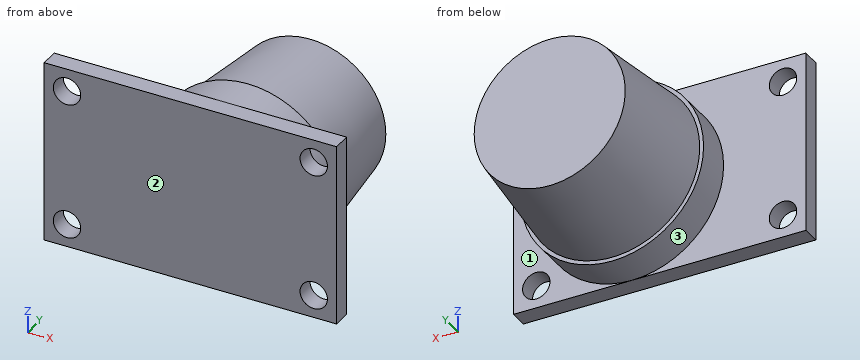
```python
from build123d import *

# Parameters (mm, degrees)
CROQUIS1_W              = 32
CROQUIS1_H              = 20
CROQUIS1_R              = 1.5
SALIENTE_EXTRUIR1_DEPTH = 2
CROQUIS2_R              = 10
SALIENTE_EXTRUIR2_DEPTH = 16.5
SALIENTE_EXTRUIR2_TAPER = 6
CROQUIS4_R              = 10
SALIENTE_EXTRUIR3_DEPTH = 4


with BuildPart() as part:
    # Croquis1 → Saliente-Extruir1 (new body)
    with BuildSketch(Plane(origin=(0, 0, 0), x_dir=(1, 0, 0), z_dir=(0, 1, 0))):
        Rectangle(CROQUIS1_W, CROQUIS1_H)
        with Locations(Location((-13.5, 7.5, 0), (0, 0, 270))):
            Circle(CROQUIS1_R, mode=Mode.SUBTRACT)
        with Locations(Location((13.5, 7.5, 0), (0, 0, 270))):
            Circle(CROQUIS1_R, mode=Mode.SUBTRACT)
        with Locations(Location((-13.5, -7.5, 0), (0, 0, 270))):
            Circle(CROQUIS1_R, mode=Mode.SUBTRACT)
        with Locations(Location((13.5, -7.5, 0), (0, 0, 270))):
            Circle(CROQUIS1_R, mode=Mode.SUBTRACT)
    extrude(amount=SALIENTE_EXTRUIR1_DEPTH)

    # Croquis2 → Saliente-Extruir2 (add)
    with BuildSketch(Plane(origin=(0, 2, 0), x_dir=(1, 0, 0), z_dir=(0, 1, 0))):
        with Locations((3, 0)):
            Circle(CROQUIS2_R)
    extrude(amount=SALIENTE_EXTRUIR2_DEPTH, taper=SALIENTE_EXTRUIR2_TAPER)

    # Croquis4 → Saliente-Extruir3 (add)
    with BuildSketch(Plane(origin=(0, 2, 0), x_dir=(1, 0, 0), z_dir=(0, 1, 0))):
        with Locations(Location((3, 0, 0), (0, 0, 270))):
            Circle(CROQUIS4_R)
    extrude(amount=SALIENTE_EXTRUIR3_DEPTH)


solid = part.part
```
Can you work these out from the model? Positions are in its coordinate system, mm. Face numbers are marked on the shaded views. A direction names the side the tool comes from. Give positions to 0.01 mm unless a question says otherwise; leave off trailing zeros. Write each loop counter-clockwise with the first axis right and the second up, starting at its lowest first coordinate (ties: lowest second). Pieces come first, ordered by that corner, then holes. Notation, with made-up numbers: (-33.75, 80) -> (11.25, 80) arc R28 cw to (11.25, 113) -> close; hole circle Ø4 at (-24, -8.5). An arc over 180 degrees is marked (long way). One line per item, written item: value.
Q1. Which directions (+Z, -Z, +X, -X, +Y, -Y) give clear straight access to the entire face, cutting with the end or side of a thin tool? Please do the marked faces 1, 2 and 3.
Results found:
face 1: +X, +Y
face 2: +Z, -Z, +X, -X, -Y
face 3: +Y
Q2. Please list where these lines run through material, in increasing order: line 1 (X direction, y = 0.95, z = -7.5); line 2 (Y direction, x = -5, z = -7.25); line 3 (Z direction, x = 6, y = 7.5). Write a range as [from, to].
Results found:
line 1: x = [-16, -15], [-12, 12], [15, 16]
line 2: y = [0, 2]
line 3: z = [-8.93, 8.93]
Q3. Imagine slicing it at B-B on z = -6.75. Give the number of separate pieces and of enclosed holes in the cut face, and give its area (3 significant figures).
Results found:
separate pieces: 3
enclosed holes: 0
area: 258 mm^2
Q4. Imagine slicing it at D-D on y = 8.5. Please give me the cut outline in (x, z).
Results found:
outline: circle Ø18.63 at (3, 0)
Q5. Imagine slicing it at C-C on x = -7.5. Please give me the cut outline in (y, z), and give its area (3 significant figures).
Results found:
outline: (0, -10) -> (2, -10) -> (2, 10) -> (0, 10) -> close
area: 40.0 mm^2
Q6. For P1, Ø5, axis at y = 5.5, z = -0.5, coming from the +X side; P2, Ø2, axis at x = 5, y = 7.5, coming from the +Z side; P3, Ø1, axis at x = -8, y = 11.5, coming from the +Z side; P4, Ø2, axis at x = 5, y = 16, coming from the -Z side, each with a flat end and sliding along its axis, tell me the tip position at first contact or that it passes through.
Results found:
P1: stops at x = 13
P2: stops at z = 9.41
P3: passes through
P4: stops at z = -8.51
Q7. Imagine slicing it at A-A on x = -13.5. Please give me the cut outline in (y, z).
Results found:
outline: (0, -10) -> (2, -10) -> (2, -9) -> (0, -9) -> close; (0, -6) -> (2, -6) -> (2, 6) -> (0, 6) -> close; (0, 9) -> (2, 9) -> (2, 10) -> (0, 10) -> close
